from build123d import *

# Parameters (mm, degrees)
SKETCH1_R           = 0.9652
BOSS_EXTRUDE1_DEPTH = 30
SKETCH2_R           = 1.8542
BOSS_EXTRUDE2_DEPTH = 1.905
CUT_EXTRUDE1_DEPTH  = 1.524


with BuildPart() as part:
    # Sketch1 → Boss-Extrude1 (new body)
    with BuildSketch(Plane.XY):
        Circle(SKETCH1_R)
    extrude(amount=BOSS_EXTRUDE1_DEPTH)

    # Sketch2 → Boss-Extrude2 (add)
    with BuildSketch(Plane.XY):
        Circle(SKETCH2_R)
    extrude(amount=-BOSS_EXTRUDE2_DEPTH)

    # Sketch3 → Cut-Extrude1 (cut)
    with BuildSketch(Plane(origin=(0, 0, -1.905), x_dir=(-1, 0, 0), z_dir=(0, 0, -1))):
        Polygon((0.850552417, 0), (0.425276208, 0.7366), (-0.425276208, 0.7366), (-0.850552417, 0), (-0.425276208, -0.7366), (0.425276208, -0.7366), align=None)
    extrude(amount=-CUT_EXTRUDE1_DEPTH, mode=Mode.SUBTRACT)


solid = part.part
Model file for the job. Use its own axes, mm. A direction names the side the tool comes from. Round coordinates to 2 decimals unless told otherwise and drop trailing zeros. Loops run counter-clockwise (first coordinate to the right, second up) from the corner with the lowest first, then second, coordinate; pieces in that order, holes last.
1. Tool access for faces 1 (the flat face through (1, -1, 0)), 2 (the flat face through (0, 0.737, -1)), 3 (the flat face through (0, -1, -1.905)): list every direction of +Z, -Z, +X, -X, +Y, -Y with a clear straight run to the whole face (end or side of a thin tool).
Check values:
face 1: +Z
face 2: -Z
face 3: -Z, +X, -X, +Y, -Y
2. Wall check: probe 1 along Z at (x, y) = (0.35, -1.25) (3 decimals); probe 2 along X at (y, z) = (0.45, 14); probe 3 along Z at (x, y) = (0.05, 0.25). Give the ranges that are in metal, low to high.
Check values:
probe 1: z = -1.905 to 0
probe 2: x = -0.85 to 0.85
probe 3: z = -0.38 to 30
3. Drop flat-ended pins along their axis: P1, Ø1.5, axis at x = 0, z = 4.5, coming from the +Y side; P2, Ø0.7, axis at x = 0.5, y = 0.5, coming from the -Z side (3 decimals). Give the stop position or say it passes through.
Check values:
P1: stops at y = 0.97
P2: stops at z = -1.905
4. Band-saw the part on B-B, the plane z = 12.5. List the corners of the cut face in (x, y).
Check values:
outline: circle Ø1.93 at (0, 0)
5. Band-saw the part on A-A, the plane x = 0. List the corners of the cut face in (y, z) (3 decimals), and give its area (3 significant figures).
Check values:
outline: (-1.854, -1.905) - (-0.737, -1.905) - (-0.737, -0.381) - (0.737, -0.381) - (0.737, -1.905) - (1.854, -1.905) - (1.854, 0) - (0.965, 0) - (0.965, 30) - (-0.965, 30) - (-0.965, 0) - (-1.854, 0) - close
area: 62.7 mm2
6. Mould opens along X. For faces 4 (the flat face through (0, 0, 30)), 5 (the cylindrical face through (-0.126, 0.957, 14.79)), 6 (the flat face through (0, -0.737, -1)) say: +X half, -X half, draft (parallel to the pull), parting line (faces both ways), or undercut.
Check values:
face 4: draft
face 5: parting line
face 6: undercut
